Autodesk Inventor part; units mm, degrees
ref_plane "Work Plane5" through (60.528, 0, 0) normal (1, 0, 0) x (0, 1, 0)
ref_plane "YZ Plane" through (0, 0, 0) normal (1, 0, 0) x (0, 1, 0)
ref_plane "XZ Plane" through (0, 0, 0) normal (0, 1, 0) x (-1, 0, 0)
sketch "Sketch4" plane through (0, 0, 0) normal (0, 1, 0) x (-1, 0, 0)
  circle A0 centre (0, 0) radius 60.528
  line L0 (-60.528, 0) -> (0, 0) construction
  circle A1 centre (0, 0) radius 52
  circle A2 centre (-60.528, 0) radius 50
  circle A3 centre (-60.528, 0) radius 40
  line L1 (-10.528, 0) -> (-20.528, 0) construction
  line L2 (-52, 0) -> (-60.528, 0) construction
  circle A4 centre (-15.528, 0) radius 3.1
  circle A5 centre (-56.264, 0) radius 3.1
  circle A6 centre (-56.264, -3.1) radius 1.65
  circle A7 centre (-56.264, 3.1) radius 1.65
  circle A8 centre (60.528, 0) radius 2.5
  circle A9 centre (-30.264, 52.4188) radius 2.5
  circle A10 centre (-30.264, -52.4188) radius 2.5
  line L3 (60.528, 0) -> (60.528, 0)
  point P0 (-39.3837, 33.9547)
  point P1 (-39.3837, -33.9547)
  point P2 (-31.9492, 41.0274)
  point P3 (-31.9492, -41.0274)
  point P4 (-28.0736, 53.6238)
  point P5 (-32.4028, 51.1243)
  point P6 (60.4764, 2.4995)
  point P7 (60.4764, -2.4995)
  point P8 (-32.4028, -51.1243)
  point P9 (-28.0736, -53.6238)
  dimension "d18" = 104
  dimension "d19" = 80
  dimension "d20" = 121.056
  dimension "d21" = 100
  dimension "d17" = 60.528
  dimension "d29" = 6.2
  dimension "d30" = 6.2
  dimension "d36" = 3.3
  dimension "d37" = 3.3
  dimension "d38" = 5
  dimension "d42" = 360
  dimension "d46" = 0
extrude "Extrusion3" add sketch "Sketch4" along normal blind 10 contours A0 A8 | A8 A0 A10 A2 A1 A9 | A9 A0 | A0 A10 | A2 A1 A3 A0 | A0 A3 A1 A2 | A3 A1 A0 | A2 A1 A3 | A4 | A5 A6 A7 picked at (59.7455, 0.5696) picked at (-29.7736, 51.7403) picked at (-29.7736, -51.7403)
ref_plane "Work Plane5" through (60.528, 0, 0) normal (1, 0, 0) x (0, 1, 0)
sketch "Sketch6" plane through (60.528, 0, 0) normal (1, 0, 0) x (0, 1, 0)
  line L0 (10, -60.528) -> (10, 60.528)
  line L1 (0, -60.528) -> (0, 60.528)
  line L2 (10, -60.528) -> (10, 60.528)
  line L3 (10, 0) -> (0, 0)
  line L4 (1.75, 5.5) -> (1.75, -5.5)
  line L5 (3.75, -7.5) -> (6.25, -7.5)
  line L6 (8.25, -5.5) -> (8.25, 5.5)
  line L7 (6.25, 7.5) -> (3.75, 7.5)
  line L8 (1.75, 7.5) -> (8.25, -7.5) construction
  line L9 (1.75, -7.5) -> (8.25, 7.5) construction
  arc A0 (6.25, -7.5) -> (8.25, -5.5) centre (6.25, -5.5) ccw
  arc A1 (1.75, -5.5) -> (3.75, -7.5) centre (3.75, -5.5) ccw
  arc A2 (8.25, 5.5) -> (6.25, 7.5) centre (6.25, 5.5) ccw
  arc A3 (3.75, 7.5) -> (1.75, 5.5) centre (3.75, 5.5) ccw
  point P0 (5, 0)
  dimension "d31" = 15
  dimension "d32" = 6.5
  dimension "d33" = 2
extrude "Extrusion4" cut sketch "Sketch6" against normal blind 45
extrude "Extrusion5" add sketch "Sketch4" along normal blind 20 contours A0 A8 | A9 A0 | A0 A10 picked at (59.7455, 0.5696) picked at (-29.7736, 51.7403) picked at (-29.7736, -51.7403)
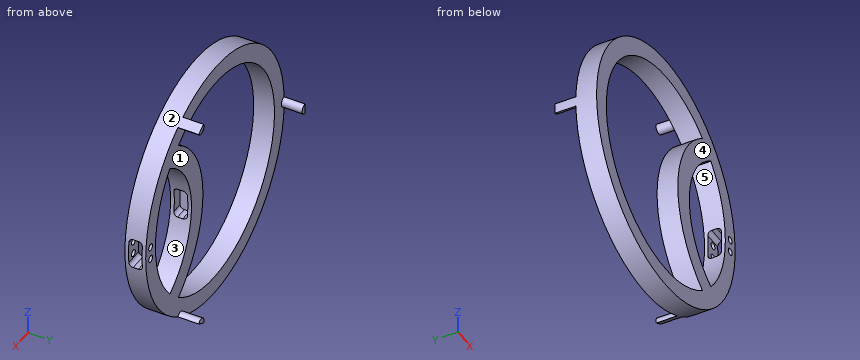
Part model, mm, in its own coordinate system. Face numbers are marked on the shaded views. A direction names the side the tool comes from. Coordinates: 2 decimals unless noted, no trailing zeros. Order: outer loops, then holes, each group sorted by start corner. A loop starts at its lowest first (then second) coordinate and runs counter-clockwise, first axis right, second up.
(1) Slice it at C-C, the plane x = 30. Write the cut outline in (y, z).
Check sheet entries:
outline: (0, -52.57) - (20, -52.57) - (20, -49.93) - (10, -49.93) - (10, -42.47) - (0, -42.47) - close; (0, -39.6) - (10, -39.6) - (10, -25.85) - (0, -25.85) - close; (0, 25.85) - (10, 25.85) - (10, 39.6) - (0, 39.6) - close; (0, 42.47) - (10, 42.47) - (10, 49.93) - (20, 49.93) - (20, 52.57) - (0, 52.57) - close
(2) Slice it at A-A, the plane x = 0. Write the cut outline in (y, z).
Check sheet entries:
outline: (0, -60.53) - (10, -60.53) - (10, -52) - (0, -52) - close; (0, 52) - (10, 52) - (10, 60.53) - (0, 60.53) - close
(3) Probe L1, parallel to Z at x = 0, y = 6; L2, parallel to X at y = 9.15, z = 3.1; L3, parallel to X at y = 2, z = -31.5. List the from-to ranges inside material, lowest first.
Check sheet entries:
L1: z = -60.53 to -52, 52 to 60.53
L2: x = -60.45 to -51.91, 10.62 to 20.65, 51.91 to 54.61, 57.91 to 60.45
L3: x = -51.69 to -41.37, 21.7 to 35.88, 41.37 to 51.69
(4) Slice it at D-D, the plane z = 43.5. Write the cut outline in (x, y), and give its area (3 significant figures).
Check sheet entries:
outline: (-42.09, 0) - (-28.49, 0) - (-28.49, 10) - (-42.09, 10) - close; (28.49, 0) - (42.09, 0) - (42.09, 10) - (28.49, 10) - close
area: 272 mm2
(5) Tool access for the marked faces 4 and 5: list every direction of +Z, -Z, +X, -X, +Y, -Y with a clear straight run to the whole face (end or side of a thin tool).
Check sheet entries:
face 4: +Z, -Z, +X, -X, -Y
face 5: +Y, -Y
(6) Pull direction X, two halves, no side cores. Call the marked faces 1, 2 and 3: pulls with the +X half, pulls with the -X half, needs draft (parallel to the pull), parting line crosses it, or undercut.
Check sheet entries:
face 1: needs draft
face 2: parting line crosses it
face 3: undercut
(7) Pin check, flat tips, straight feed: pin 1 Ø10 at (x, y) = (45.5, 9.5) entering from +Z; pin 2 Ø12 at (x, y) = (-24.5, 11.5) entering from -Z; pin 3 Ø2 at (x, y) = (55, 5.5) entering from -Z; pin 4 Ø4 at (x, z) = (56.264, -3.1) entering from -Y. Stop position of each tip, or through.
Check sheet entries:
pin 1: stops at z = 44.98
pin 2: stops at z = -57.57
pin 3: stops at z = -27.34
pin 4: stops at y = 0
(8) Slice it at B-B, the plane z = -14. Write the cut outline in (x, y).
Check sheet entries:
outline: (-58.89, 0) - (-50.08, 0) - (-50.08, 10) - (-58.89, 10) - close; (12.53, 0) - (23.06, 0) - (23.06, 10) - (12.53, 10) - close; (50.08, 0) - (58.89, 0) - (58.89, 10) - (50.08, 10) - close
